Can you work these out from the model? Positions are in its coordinate system, mm. A direction names the side the tool comes from. Round coordinates to 2 decimals unless told otherwise and drop trailing zeros. Write each loop counter-clockwise with the first axis right and the second up, starting at its lowest first coordinate (ties: lowest second). Pieces come first, ordered by that corner, then holes. Notation, with made-up numbers: (60.5, -19.75) -> (102.5, -19.75) arc R21 cw to (102.5, -11.75) -> close; hole circle Ø8 at (-6.5, 36). An arc over 180 degrees is marked (long way). Write item = value, one per line. Start each with the question number.
1) If I drill on line 1 (Z direction, x = 126, y = 0.5); line 2 (Y direction, x = 144.5, z = 6.75); line 3 (Y direction, x = 90, z = 0), over which ranges is the centre line in solid material (lowest first)?
2) I'm going to push flat-ended pins straight in: pin 1 (4.5 mm diameter, centred on x = 86.5, y = 0, fed in from -Z); pin 2 (2 mm diameter, centred on x = 145, y = 0.5, fed in from +Z); pin 3 (2 mm diameter, centred on x = 123, z = 0, fed in from +Y). Where does each tip first touch, or does it pass through?
3) For faces 4 (the face through (123, 0, 3.9)), 5 (the face through (123, 0, -3.9)), 6 (the face through (123, 3.9, 0)), 7 (the face through (0, 2, -2)), which set-ups out of +Z, -Z, +X, -X, +Y, -Y let a thin tool reach every point of the face, with its end or its side?
4) Imagine slicing it at A-A, the plane z = 0. Please give me the cut outline in (x, y), then the cut area to 3 significant figures.
5) Thinking about a two-plate mould opening in Z: for faces 1 (the face through (123, -3.9, 0)), 2 (the face through (123, 7, 10)), 3 (the face through (123, 10, 7)), which applies, +Z half, -Z half, draft (parallel to the pull), parting line (faces both ways), or undercut?
from build123d import *

# Parameters (mm, degrees)
SKETCH1_W                = 20
SKETCH1_H                = 20
BOSS_EXTRUDE1_DEPTH      = 250
FILLET1_R                = 1
CUT_EXTRUDE1_DEPTH       = 251.399680511
F_5_0_5_DIAMETER_HOLE1_D = 5
FILLET2_R                = 2
FILLET3_R                = 0.5
FILLET4_R                = 0.5
FILLET5_R                = 0.5


with BuildPart() as part:
    # Sketch1 → Boss-Extrude1 (new body)
    with BuildSketch(Plane(origin=(0, 0, 0), x_dir=(0, 0, -1), z_dir=(1, 0, 0))):
        Rectangle(SKETCH1_W, SKETCH1_H)
    extrude(amount=BOSS_EXTRUDE1_DEPTH)

    # Fillet1
    fillet1_edges = [part.edges().sort_by_distance(p)[0] for p in [
        (125, 10, 10),
        (125, 10, -10),
        (125, -10, -10),
        (125, -10, 10),
    ]]
    fillet(fillet1_edges, radius=FILLET1_R)

    # Sketch3 → Cut-Extrude1 (cut, through all)
    with BuildSketch(Plane.ZY):
        Polygon((-3.6, 10), (3.6, 10), (3.6, 9.5), (3.1, 9.5), (3.1, 8.2), (5.63, 8.2), (5.63, 6.619949494), (2.910050506, 3.9), (-2.910050506, 3.9), (-5.63, 6.619949494), (-5.63, 8.2), (-3.1, 8.2), (-3.1, 9.5), (-3.6, 9.5), align=None)
        Polygon((10, 3.6), (10, -3.6), (9.5, -3.6), (9.5, -3.1), (8.2, -3.1), (8.2, -5.63), (6.619949494, -5.63), (3.9, -2.910050506), (3.9, 2.910050506), (6.619949494, 5.63), (8.2, 5.63), (8.2, 3.1), (9.5, 3.1), (9.5, 3.6), align=None)
        Polygon((3.6, -10), (-3.6, -10), (-3.6, -9.5), (-3.1, -9.5), (-3.1, -8.2), (-5.63, -8.2), (-5.63, -6.619949494), (-2.910050506, -3.9), (2.910050506, -3.9), (5.63, -6.619949494), (5.63, -8.2), (3.1, -8.2), (3.1, -9.5), (3.6, -9.5), align=None)
        Polygon((-10, -3.6), (-10, 3.6), (-9.5, 3.6), (-9.5, 3.1), (-8.2, 3.1), (-8.2, 5.63), (-6.619949494, 5.63), (-3.9, 2.910050506), (-3.9, -2.910050506), (-6.619949494, -5.63), (-8.2, -5.63), (-8.2, -3.1), (-9.5, -3.1), (-9.5, -3.6), align=None)
    extrude(amount=-CUT_EXTRUDE1_DEPTH, mode=Mode.SUBTRACT)

    # Ø5.0 (5) Diameter Hole1 (through all)
    with Locations(Plane.ZY):
        with Locations((0, 0)):
            Hole(F_5_0_5_DIAMETER_HOLE1_D / 2)

    # Fillet2
    fillet2_edges = [part.edges().sort_by_distance(p)[0] for p in [
        (125, -3.9, -2.910050506),
        (125, -3.9, 2.910050506),
        (125, 2.910050506, -3.9),
        (125, -2.910050506, -3.9),
        (125, -2.910050506, 3.9),
        (125, 2.910050506, 3.9),
        (125, 3.9, 2.910050506),
        (125, 3.9, -2.910050506),
    ]]
    fillet(fillet2_edges, radius=FILLET2_R)

    # Fillet3
    fillet3_edges = [part.edges().sort_by_distance(p)[0] for p in [
        (125, 3.6, -10),
        (125, 3.1, -9.5),
        (125, 3.1, -8.2),
        (125, 5.63, -8.2),
        (125, 5.63, -6.619949494),
        (125, 3.6, 10),
        (125, 3.1, 9.5),
        (125, 3.1, 8.2),
        (125, 5.63, 8.2),
        (125, 5.63, 6.619949494),
        (125, 6.619949494, 5.63),
        (125, 8.2, 5.63),
        (125, 8.2, 3.1),
        (125, 9.5, 3.1),
        (125, 10, 3.6),
        (125, 9.5, -3.1),
        (125, 10, -3.6),
        (125, 8.2, -3.1),
        (125, 8.2, -5.63),
        (125, 6.619949494, -5.63),
    ]]
    fillet(fillet3_edges, radius=FILLET3_R - 0.0001)  # a hair under: the kernel refuses the full size

    # Fillet4
    fillet4_edges = [part.edges().sort_by_distance(p)[0] for p in [
        (125, -3.6, 10),
        (125, -3.1, 9.5),
        (125, -3.1, 8.2),
        (125, -5.63, 8.2),
        (125, -5.63, 6.619949494),
        (125, -6.619949494, 5.63),
        (125, -8.2, 5.63),
        (125, -8.2, 3.1),
        (125, -10, 3.6),
        (125, -9.5, 3.1),
        (125, -10, -3.6),
        (125, -9.5, -3.1),
        (125, -8.2, -3.1),
        (125, -8.2, -5.63),
        (125, -6.619949494, -5.63),
        (125, -5.63, -6.619949494),
        (125, -5.63, -8.2),
        (125, -3.1, -8.2),
        (125, -3.1, -9.5),
        (125, -3.6, -10),
    ]]
    fillet(fillet4_edges, radius=FILLET4_R - 0.0001)  # a hair under: the kernel refuses the full size

    # Fillet5
    fillet5_edges = [part.edges().sort_by_distance(p)[0] for p in [
        (125, 3.6, 9.5),
        (125, 9.5, 3.6),
        (125, 9.5, -3.6),
        (125, 3.6, -9.5),
        (125, -3.6, 9.5),
        (125, -9.5, 3.6),
        (125, -9.5, -3.6),
        (125, -3.6, -9.5),
    ]]
    fillet(fillet5_edges, radius=FILLET5_R)


solid = part.part
Reported:
q1.line_1 = -3.9 to -2.45, 2.45 to 3.9
q1.line_2 = -10 to -5.62, 5.62 to 10
q1.line_3 = -3.9 to -2.5, 2.5 to 3.9
q2.pin_1 = -3.91
q2.pin_2 = 3.9
q2.pin_3 = 3.9
q3.face_4 = +Z, +X, -X
q3.face_5 = -Z, +X, -X
q3.face_6 = +X, -X, +Y
q3.face_7 = +Z, -Z, -X, +Y, -Y
q4.outline = (0, -3.9) -> (250, -3.9) -> (250, -2.5) -> (0, -2.5) -> close; (0, 2.5) -> (250, 2.5) -> (250, 3.9) -> (0, 3.9) -> close
q4.area = 700 mm²
q5.face_1 = undercut
q5.face_2 = +Z half
q5.face_3 = draft
